For this review, use the dimensioned drawing (mm, ordinates from the lowest corner) and the shaded views. A direction names the side the tool comes from. Give positions to 0.01 mm unless a question says otherwise; leave off trailing zeros. Loops run counter-clockwise (first coordinate to the right, second up) from the corner with the lowest first, then second, coordinate; pieces in that order, holes last. Notation, with made-up numbers: (62.25, 13) - (69.25, 13) arc R9 ccw to (69.25, 28) - close; hole circle Ø11 at (61, -10). An arc over 180 degrees is marked (long way). Write each question's results on one line, items separated by ' | '.
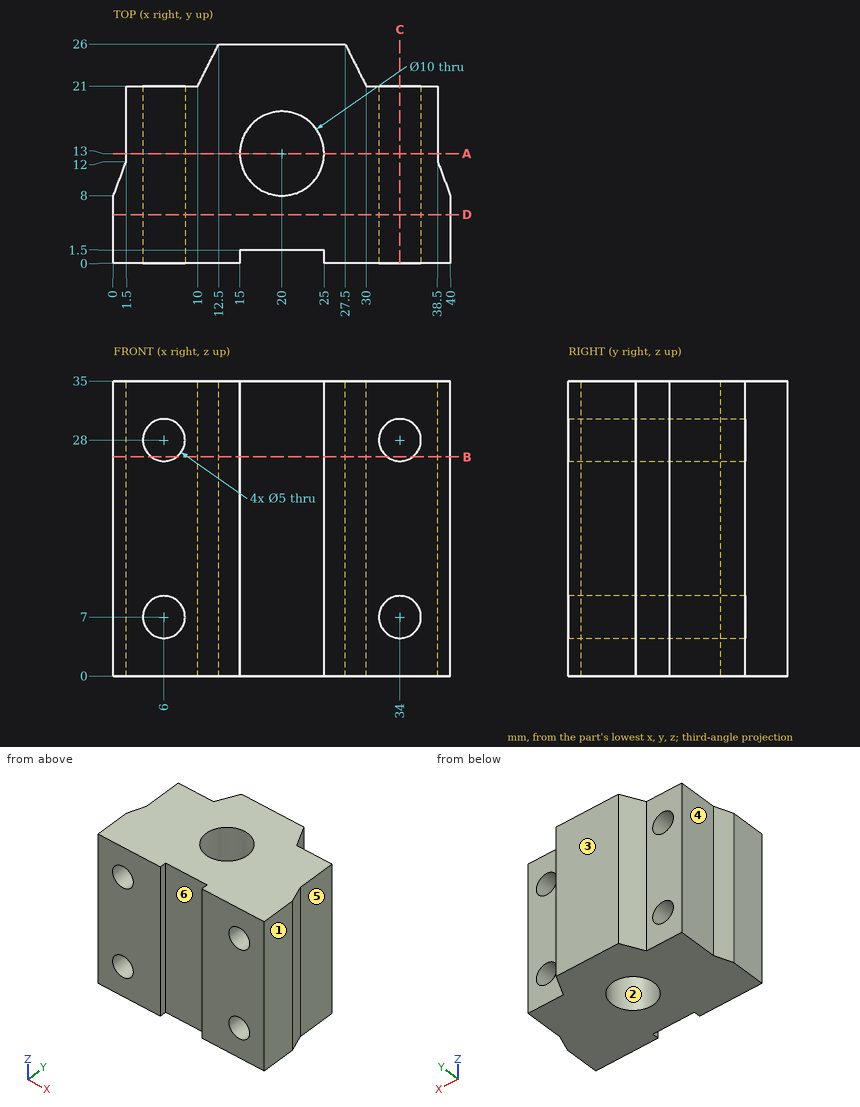
Item 1: We need section B-B on z = 26. Give the boundary of the cut face in (x, y).
Output values:
outline: (0, 0) - (4.5, 0) - (4.5, 21) - (1.5, 21) - (1.5, 12) - (0, 8) - close; (7.5, 0) - (15, 0) - (15, 1.5) - (25, 1.5) - (25, 0) - (32.5, 0) - (32.5, 21) - (30, 21) - (27.5, 26) - (12.5, 26) - (10, 21) - (7.5, 21) - close; (35.5, 0) - (40, 0) - (40, 8) - (38.5, 12) - (38.5, 21) - (35.5, 21) - close; hole circle Ø10 at (20, 13)
Item 2: We need section C-C on x = 34. Give the boundary of the cut face in (y, z), then the cut area to 3 significant figures.
Output values:
outline: (0, 0) - (21, 0) - (21, 4.5) - (0, 4.5) - close; (0, 9.5) - (21, 9.5) - (21, 25.5) - (0, 25.5) - close; (0, 30.5) - (21, 30.5) - (21, 35) - (0, 35) - close | area: 525 mm²
Item 3: We need section D-D on y = 5.75. Give the boundary of the cut face in (x, z), then the cut area to 3 significant figures.
Output values:
outline: (0, 0) - (40, 0) - (40, 35) - (0, 35) - close; hole circle Ø5 at (6, 7); hole circle Ø5 at (6, 28); hole circle Ø5 at (34, 7); hole circle Ø5 at (34, 28) | area: 1,320 mm²
Item 4: Clearance check with flat-ended pins moving along their axes: P1, Ø3, axis at y = 21, z = 20.5, coming from the -X side; P2, Ø7, axis at y = 18, z = 17, coming from the +X side; P3, Ø3, axis at x = 34, z = 7, coming from the +Y side; P4, Ø6.5, axis at x = 34, z = 28, coming from the +Y side. State where each tip first meets the part, or that it passes through.
Output values:
P1: stops at x = 1.5 | P2: stops at x = 38.5 | P3: passes through | P4: stops at y = 21
Item 5: Wall thickness on probe 1 along X at (y, z) = (2, 28); probe 2 along X at (y, z) = (8.75, 28); probe 3 along Y at (x, z) = (20, 24): over which ranges is each line inside the solid? List them lowest first.
Output values:
probe 1: x = 0 to 3.5, 8.5 to 31.5, 36.5 to 40 | probe 2: x = 0.28 to 3.5, 8.5 to 17.37, 22.63 to 31.5, 36.5 to 39.72 | probe 3: y = 1.5 to 8, 18 to 26
Item 6: Tool access review of the marked faces 4, 5 and 6: name each direction out of +Z, -Z, +X, -X, +Y, -Y from which nothing blocks a thin tool from reaching the whole face with its end or side.
Output values:
face 4: +Z, -Z, -X, +Y | face 5: +Z, -Z, +X, +Y | face 6: +Z, -Z, -Y
Item 7: We need section A-A on y = 13. Give the boundary of the cut face in (x, z).
Output values:
outline: (1.5, 0) - (15, 0) - (15, 35) - (1.5, 35) - close; (25, 0) - (38.5, 0) - (38.5, 35) - (25, 35) - close; hole circle Ø5 at (6, 7); hole circle Ø5 at (6, 28); hole circle Ø5 at (34, 7); hole circle Ø5 at (34, 28)
Item 8: Draft analysis for pull direction X (two halves, no side actions). For the marked faces 1, 2 and 3, state which applies: +X half, -X half, draft (parallel to the pull), parting line (faces both ways), or undercut.
Output values:
face 1: +X half | face 2: undercut | face 3: draft
